```python
from build123d import *

# Parameters (mm, degrees)
F0_W     = 215.9
F0_H     = 76.2
F1_DEPTH = 6.35
F3_DEPTH = 6.35


with BuildPart() as f1:
    # F0 (on Front) → F1 (new body)
    with BuildSketch(Plane.XZ):
        with Locations((4.005505, 0.249261)):
            Rectangle(F0_W, F0_H)
    extrude(amount=F1_DEPTH)

    # F2 (on face) → F3 (join)
    with BuildSketch(Plane.XZ.offset(6.35)):
        Polygon((-103.944495, 0), (-143.752261, 0), (-143.752261, -38.1), (148.347739, -38.1), (148.347739, 0), (111.955505, 0), (111.955505, -37.850739), (-103.944495, -37.850739), align=None)
    extrude(amount=-F3_DEPTH)


solid = f1.part
```
For this review, take the finished solid that the model builds, in its own axes (mm). A direction names the side the tool comes from. Give positions to 0.01 mm unless a question says otherwise; leave off trailing zeros. Write each loop counter-clockwise with the first axis right and the second up, starting at its lowest first coordinate (ties: lowest second). Pieces come first, ordered by that corner, then holes. Notation, with made-up numbers: M 44.25,72.25 L 81.25,72.25 A21 cw 81.25,110.25 Z; hole C -15,49.25 d11. An arc over 180 degrees is marked long. Answer as a JSON object with one key per item and string values. Group by question number.
Item 1: For pin 1 Ø1.9 at (x, y) = (-129.5, -2) entering from +Z; pin 2 Ø1.5 at (x, z) = (42.5, 22.5) entering from +Y, all flat-tipped, find the tip position at first contact; note any pin that passes through.
Item 2: For probe 1 along X at (y, z) = (-5, 26); probe 2 along Z at (x, y) = (125.5, -5.5), list the stretches that pass through material, from the lowest coordinate up. Write a range as [from, to].
Item 3: Tool access review of faces 1 (the flat face through (0, 0, 1)), 2 (the flat face through (-124, -3, 0)), 3 (the flat face through (111.956, -3, 19)): name each direction out of +Z, -Z, +X, -X, +Y, -Y from which nothing blocks a thin tool from reaching the whole face with its end or side.
Item 4: Consider section A-A on y = -2.75. Write out the cut boundary in (x, z), plus the area to 3 significant figures.
Item 5: Consider section B-B on x = -111. Write out the cut boundary in (y, z).
Item 6: Consider section C-C on z = 9.5. Write out the cut boundary in (x, y), plus the area to 3 significant figures.
Check result:
{
 "1": {"pin 1": "stops at z = 0", "pin 2": "stops at y = 0"},
 "2": {"probe 1": "x = [-103.94, 111.96]", "probe 2": "z = [-38.1, 0]"},
 "3": {"face 1": "+Z, -Z, +X, -X, +Y", "face 2": "+Z, -X, +Y, -Y", "face 3": "+Z, +X, +Y, -Y"},
 "4": {"outline": "M -143.75,-38.1 L 148.35,-38.1 L 148.35,0 L 111.96,0 L 111.96,38.35 L -103.94,38.35 L -103.94,0 L -143.75,0 Z", "area": "19,400 mm^2"},
 "5": {"outline": "M -6.35,-38.1 L 0,-38.1 L 0,0 L -6.35,0 Z"},
 "6": {"outline": "M -103.94,-6.35 L 111.96,-6.35 L 111.96,0 L -103.94,0 Z", "area": "1,370 mm^2"}
}
